Read the model definition and answer for the solid it produces. Units are mm, in the model's axes. A direction names the side the tool comes from. Coordinates: 2 decimals unless noted, no trailing zeros. Loops run counter-clockwise (first coordinate to the right, second up) from the corner with the lowest first, then second, coordinate; pieces in that order, holes last. Notation, with made-up numbers: (-6, 24) -> (7, 24) arc R12 cw to (7, 44) -> close; hole circle Ø10 at (54.25, -7.75). An arc over 180 degrees is marked (long way). Answer as a JSON object with one key per item and string values. Group by question number.
Q1. Each of these flat-tipped pins is pushed along its axis until it touches: P1, Ø2, axis at x = 0, z = -62, coming from the -Y side; P2, Ø12, axis at x = 57.5, z = -59.5, coming from the +Y side; P3, Ø3, axis at x = -63.5, z = -12.7, coming from the +Y side. Where does it stop, or does it pass through?
Q2. The part is cut by section C-C on z = -88.9. Write down the section's boundary in (x, y) (3 decimals), and give its area (3 significant figures).
Q3. The part is cut by section D-D on x = -0.5. Write down the section's boundary in (y, z).
Q4. The part is cut by section A-A on y = 27. Write down the section's boundary in (x, z) (3 decimals).
Q5. The part is cut by section B-B on x = -63.5. Write down the section's boundary in (y, z).
Q6. Straight lines are drawn through the part: line 1 along Z through (x, y) = (63.5, 19.75); line 2 along X through (y, z) = (19.75, -12.7); line 3 along X through (y, z) = (22, -12). For each, find the intervals that lie inside material, in ascending order. Write a range as [from, to].
Q7. Determine the mould class of faces 1 (the flat face through (73.025, -29, -50)), 2 (the flat face through (76.2, 0, -50)), 3 (the flat face through (-1, 0, 0)), 4 (the flat face through (63, 15.4, -89)) for opening direction X: released by +X, released by -X, zero draft, split by the parting line, or undercut.
Q8. For faces 5 (the flat face through (-1, 25.4, -51)), 6 (the flat face through (-1, -25.4, -51)), 7 (the flat face through (-76.2, 0, -50)), determine the directions among +Z, -Z, +X, -X, +Y, -Y from which every point of the face is accessible in a straight line to the end or side of a thin tool.
from build123d import *

# Parameters (mm, degrees)
SKETCH1_W           = 152.4
SKETCH1_H           = 63.5
BOSS_EXTRUDE1_DEPTH = 101.6
SKETCH3_W           = 146.05
SKETCH3_H           = 95.34
CUT_EXTRUDE1_DEPTH  = 6.35
SKETCH4_R           = 1.78
CUT_EXTRUDE2_DEPTH  = 10


with BuildPart() as part:
    # Sketch1 → Boss-Extrude1 (new body)
    with BuildSketch(Plane.XY):
        Rectangle(SKETCH1_W, SKETCH1_H)
    extrude(amount=-BOSS_EXTRUDE1_DEPTH)

    # Sketch3 → Cut-Extrude1 (cut)
    with BuildSketch(Plane(origin=(0, 31.75, 0), x_dir=(1, 0, 0), z_dir=(0, 1, 0))):
        with Locations((0, 50.8)):
            Rectangle(SKETCH3_W, SKETCH3_H)
    cut_extrude1 = extrude(amount=-CUT_EXTRUDE1_DEPTH, mode=Mode.SUBTRACT)

    # Mirror1: Cut-Extrude1 across plane
    add(cut_extrude1.mirror(Plane.ZX), mode=Mode.SUBTRACT)

    # Sketch4 → Cut-Extrude2 (cut)
    with BuildSketch(Plane(origin=(0, 25.4, 0), x_dir=(1, 0, 0), z_dir=(0, 1, 0))):
        with Locations((63.5, 88.9)):
            Circle(SKETCH4_R)
        with Locations((63.5, 12.7)):
            Circle(SKETCH4_R)
        with Locations((-63.5, 88.9)):
            Circle(SKETCH4_R)
        with Locations((-63.5, 12.7)):
            Circle(SKETCH4_R)
    extrude(amount=-CUT_EXTRUDE2_DEPTH, mode=Mode.SUBTRACT)


solid = part.part
Final values:
{
 "1": {"P1": "stops at y = -25.4", "P2": "stops at y = 25.4", "P3": "stops at y = 15.4"},
 "2": {"outline": "(-76.2, -31.75) -> (-73.025, -31.75) -> (-73.025, -25.4) -> (73.025, -25.4) -> (73.025, -31.75) -> (76.2, -31.75) -> (76.2, 31.75) -> (73.025, 31.75) -> (73.025, 25.4) -> (65.28, 25.4) -> (65.28, 15.4) -> (61.72, 15.4) -> (61.72, 25.4) -> (-61.72, 25.4) -> (-61.72, 15.4) -> (-65.28, 15.4) -> (-65.28, 25.4) -> (-73.025, 25.4) -> (-73.025, 31.75) -> (-76.2, 31.75) -> close", "area": "7,750 mm2"},
 "3": {"outline": "(-31.75, -101.6) -> (31.75, -101.6) -> (31.75, -98.47) -> (25.4, -98.47) -> (25.4, -3.13) -> (31.75, -3.13) -> (31.75, 0) -> (-31.75, 0) -> (-31.75, -3.13) -> (-25.4, -3.13) -> (-25.4, -98.47) -> (-31.75, -98.47) -> close"},
 "4": {"outline": "(-76.2, -101.6) -> (76.2, -101.6) -> (76.2, 0) -> (-76.2, 0) -> close; hole (-73.025, -98.47) -> (73.025, -98.47) -> (73.025, -3.13) -> (-73.025, -3.13) -> close"},
 "5": {"outline": "(-31.75, -101.6) -> (31.75, -101.6) -> (31.75, -98.47) -> (25.4, -98.47) -> (25.4, -90.68) -> (15.4, -90.68) -> (15.4, -87.12) -> (25.4, -87.12) -> (25.4, -14.48) -> (15.4, -14.48) -> (15.4, -10.92) -> (25.4, -10.92) -> (25.4, -3.13) -> (31.75, -3.13) -> (31.75, 0) -> (-31.75, 0) -> (-31.75, -3.13) -> (-25.4, -3.13) -> (-25.4, -98.47) -> (-31.75, -98.47) -> close"},
 "6": {"line 1": "z = [-101.6, -90.68], [-87.12, -14.48], [-10.92, 0]", "line 2": "x = [-76.2, -65.28], [-61.72, 61.72], [65.28, 76.2]", "line 3": "x = [-76.2, -65.14], [-61.86, 61.86], [65.14, 76.2]"},
 "7": {"face 1": "undercut", "face 2": "released by +X", "face 3": "zero draft", "face 4": "undercut"},
 "8": {"face 5": "+Y", "face 6": "-Y", "face 7": "+Z, -Z, -X, +Y, -Y"}
}
